Design review of the part built by this model. Coordinates are the model's own, in mm. A direction names the side the tool comes from. Give positions to 0.01 mm unless a question says otherwise; leave off trailing zeros. Order: outer loops, then holes, each group sorted by start corner. A loop starts at its lowest first (then second) coordinate and runs counter-clockwise, first axis right, second up. Notation, with made-up numbers: M -16.5,64 L -3.5,64 A13 cw -3.5,76 Z; hole C 6.25,84.25 d1. An arc over 180 degrees is marked long. Put each result on its own line as item: value. Start each with the question number.
from build123d import *

# Parameters (mm, degrees)
SKETCH1_R           = 18
SKETCH1_R_2         = 19
BOSS_EXTRUDE1_DEPTH = 10
SKETCH1_3_R         = 18
BOSS_EXTRUDE2_DEPTH = 212
SKETCH2_R           = 13
CUT_EXTRUDE1_DEPTH  = 200
SKETCH3_R           = 13
SKETCH3_R_2         = 12
BOSS_EXTRUDE3_DEPTH = 10


with BuildPart() as part:
    # Sketch1 → Boss-Extrude1 (new body)
    with BuildSketch(Plane.XY):
        Circle(SKETCH1_R)
        Circle(SKETCH1_R_2)
        Circle(SKETCH1_R, mode=Mode.SUBTRACT)
    extrude(amount=BOSS_EXTRUDE1_DEPTH)

    # Sketch1_3 → Boss-Extrude2 (add)
    with BuildSketch(Plane.XY):
        Circle(SKETCH1_3_R)
    extrude(amount=BOSS_EXTRUDE2_DEPTH)

    # Sketch2 → Cut-Extrude1 (cut)
    with BuildSketch(Plane.XY.offset(212)):
        Circle(SKETCH2_R)
    extrude(amount=-CUT_EXTRUDE1_DEPTH, mode=Mode.SUBTRACT)

    # Sketch3 → Boss-Extrude3 (add)
    with BuildSketch(Plane.XY.offset(212)):
        Circle(SKETCH3_R)
        Circle(SKETCH3_R_2, mode=Mode.SUBTRACT)
    extrude(amount=-BOSS_EXTRUDE3_DEPTH)


solid = part.part
1. Consider section B-B on z = 114. Give the boundary of the cut face in (x, y), then the cut area to 3 significant figures.
2. Consider section D-D on y = -15.5. Give the boundary of the cut face in (x, z).
3. Consider section A-A on x = 0. Give the boundary of the cut face in (y, z).
4. To check wall thickness, follow probe 1 along Y at (x, z) = (0, 136); probe 2 along Z at (x, y) = (-6, -8.5); probe 3 along X at (y, z) = (6, 145.5). State the ranges of each line that lie inside material, in increasing order.
5. The part is to be moulded in two halves that separate along Z. For faces 1 (the cylindrical face through (-2.343, 17.847, 109.586)), 2 (the flat face through (9, -9, 202)), 3 (the flat face through (0, 0, 0)), say which applies: +Z half, -Z half, draft (parallel to the pull), parting line (faces both ways), or undercut.
6. Insertion check: pin 1 (2 mm diameter, centred on x = 7.5, y = -8, fed in from +Z); pin 2 (4 mm diameter, centred on x = -15, z = 89, fed in from +Y); pin 3 (3 mm diameter, centred on y = 12.5, z = 33, fed in from -X). Each pin has a flat end and moves straight along its axis. Give the tip position at first contact, or say it passes through.
7. Machinability: for faces 4 (the flat face through (7, -17, 10)), 5 (the flat face through (0, 0, 12)), 6 (the cylindrical face through (8.767, -16.856, 4.93)), which of the approach directions +Z, -Z, +X, -X, +Y, -Y give a long, thin tool a straight path to every point of the face, cutting with its end or side? Answer none if there is none.
Returned:
1. outline: C 0,0 d36; hole C 0,0 d26
1. area: 487 mm2
2. outline: M -10.99,0 L 10.99,0 L 10.99,10 L 9.15,10 L 9.15,212 L -9.15,212 L -9.15,10 L -10.99,10 Z
3. outline: M -19,0 L 19,0 L 19,10 L 18,10 L 18,212 L 12,212 L 12,202 L 13,202 L 13,12 L -13,12 L -13,202 L -12,202 L -12,212 L -18,212 L -18,10 L -19,10 Z
4. probe 1: y = -18 to -13, 13 to 18
4. probe 2: z = 0 to 12
4. probe 3: x = -16.97 to -11.53, 11.53 to 16.97
5. face 1: draft
5. face 2: undercut
5. face 3: -Z half
6. pin 1: stops at z = 12
6. pin 2: stops at y = 12.45
6. pin 3: stops at x = -14.25
7. face 4: +Z
7. face 5: none
7. face 6: +Z, -Z
